Can you work these out from the drawing? Everything is in mm from the part's minimum corner. A direction names the side the tool comes from. Coordinates: 2 decimals unless noted, no trailing zeros. Loops run counter-clockwise (first coordinate to the right, second up) from the corner with the lowest first, then second, coordinate; pieces in that order, holes last. Notation, with made-up numbers: (13.25, 0.5) - (35.25, 0.5) arc R29 ccw to (35.25, 27.5) - close; hole circle Ø6 at (33, 51). An arc over 180 degrees is marked (long way). One line per question, with ' | ' between items. Start each with the question number.
1. I want a section at B-B, the plane x = 6. Write out the boundary of the cut face in (y, z).
2. Which directions (+Z, -Z, +X, -X, +Y, -Y) give clear straight access to the entire face, cutting with the end or side of a thin tool? Please do the marked faces 1, 2 and 3.
3. Please list where these lines run through material, in increasing order: L1, parallel to Z at x = 6, y = 5; L2, parallel to Y at x = 9.75, z = 8.5; L3, parallel to X at y = 1.75, z = 7.5. Write a range as [from, to].
4. I want a section at A-A, the plane z = 6. Write out the boundary of the cut face in (x, y), then the cut area to 3 significant figures.
5. I want a section at C-C, the plane z = 2.25. Write out the boundary of the cut face in (x, y).
6. I'm going to push flat-ended pins straight in: P1, Ø5, axis at x = 5.5, y = 8.5, coming from the +Z side; P2, Ø4, axis at x = 10, y = 7, coming from the -Z side; P3, Ø1, axis at x = 5.5, z = 5, coming from the -Y side; P4, Ø1, axis at y = 11, z = 3, coming from the -X side. Where does each tip first touch, or does it pass through?
7. I want a section at D-D, the plane y = 12. Write out the boundary of the cut face in (x, z).
8. We'd pull the mould along Z, two halves only. Please class the marked faces 4, 5 and 6: pulls with the +Z half, pulls with the -Z half, needs draft (parallel to the pull), parting line crosses it, or undercut.
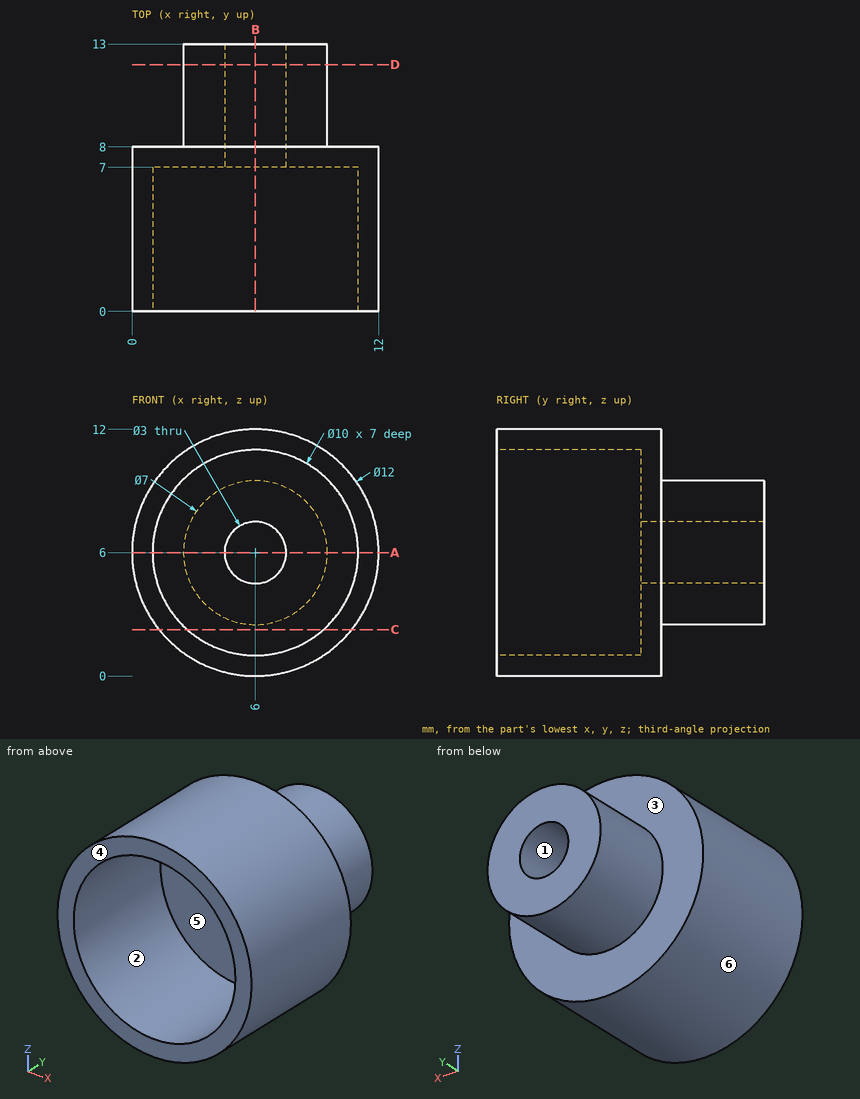
Results are:
1) outline: (0, 0) - (8, 0) - (8, 2.5) - (13, 2.5) - (13, 4.5) - (7, 4.5) - (7, 1) - (0, 1) - close; (0, 11) - (7, 11) - (7, 7.5) - (13, 7.5) - (13, 9.5) - (8, 9.5) - (8, 12) - (0, 12) - close
2) face 1: +Y, -Y | face 2: -Y | face 3: +Y
3) L1: z = [0, 1], [11, 12] | L2: y = [7, 8] | L3: x = [0.19, 1.23], [10.77, 11.81]
4) outline: (0, 0) - (1, 0) - (1, 7) - (4.5, 7) - (4.5, 13) - (2.5, 13) - (2.5, 8) - (0, 8) - close; (7.5, 7) - (11, 7) - (11, 0) - (12, 0) - (12, 8) - (9.5, 8) - (9.5, 13) - (7.5, 13) - close | area: 43.0 mm2
5) outline: (1.32, 0) - (2.69, 0) - (2.69, 7) - (9.31, 7) - (9.31, 0) - (10.68, 0) - (10.68, 8) - (1.32, 8) - close
6) P1: stops at z = 12 | P2: stops at z = 0.34 | P3: stops at y = 7 | P4: stops at x = 3.55
7) outline: circle Ø7 at (6, 6); hole circle Ø3 at (6, 6)
8) face 4: needs draft | face 5: undercut | face 6: parting line crosses it
